Check sheet for the modelled part. Datum: model origin and axes. Units: mm. Give positions to 0.01 mm unless a question says otherwise; leave off trailing zeros. Loops run counter-clockwise (first coordinate to the right, second up) from the corner with the lowest first, then second, coordinate; pieces in that order, holes last. Notation, with made-up numbers: (-3, 83) -> (20, 83) arc R21 cw to (20, 121) -> close; hole circle Ø7 at (-35.5, -7). An arc over 180 degrees is marked (long way). Write each question's results on one line, items separated by ' | '. Start each with the question number.
1. Gauge pin test, flat ends, axial feed: pin 1 Ø1.4 at (y, z) = (37.5, 3) entering from -X; pin 2 Ø1.4 at (y, z) = (36, 2) entering from +X; pin 3 Ø1.4 at (x, z) = (157.5, 1.5) entering from -Y (3 decimals). Record the tip position at first contact, or that the pin passes through.
2. Cross-section at B-B on y = 34.5. Record the boundary of the cut face in (x, z).
3. Material ranges on L1, parallel to X at y = 16, z = 3.85; L2, parallel to Y at x = 154.5, z = 0.3; L3, parallel to X at y = 5, z = 2.5, recorded low to high. Write a range as from..to.
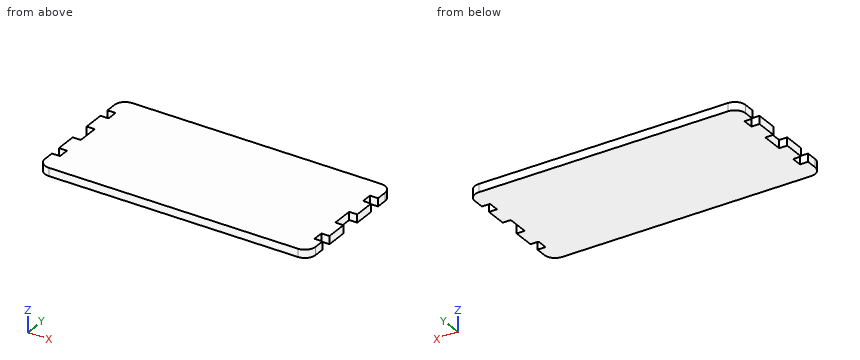
from build123d import *

# Parameters (mm, degrees)
F1_DEPTH = 4.7625


# Not quite as in the source:
# - a length typed as a fraction of an inch, garbled in the dataset ("3 / 203.2 mm" for 3/8 in), is restored
# - a feature names something its author has since deleted; it is built from what else it names


with BuildPart() as f1:
    # F0 (on Top) → F1 (new body)
    with BuildSketch(Plane.XY):
        with BuildLine():
            ThreePointArc((0, 6.35), (1.8598719395, 1.8598719395), (6.35, 0))
            Line((6.35, 0), (80.01, 0))
            Line((80.01, 0), (153.67, 0))
            ThreePointArc((153.67, 0), (158.1601280605, 1.8598719395), (160.02, 6.35))
            Line((160.02, 6.35), (160.02, 12.7))
            Line((160.02, 12.7), (155.2575, 12.7))
            Line((155.2575, 12.7), (155.2575, 19.05))
            Line((155.2575, 19.05), (160.02, 19.05))
            Line((160.02, 19.05), (160.02, 31.75))
            Line((160.02, 31.75), (155.2575, 31.75))
            Line((155.2575, 31.75), (155.2575, 44.45))
            Line((155.2575, 44.45), (160.02, 44.45))
            Line((160.02, 44.45), (160.02, 57.15))
            Line((160.02, 57.15), (155.2575, 57.15))
            Line((155.2575, 57.15), (155.2575, 63.5))
            Line((155.2575, 63.5), (160.02, 63.5))
            Line((160.02, 63.5), (160.02, 69.85))
            ThreePointArc((160.02, 69.85), (158.1601280605, 74.3401280605), (153.67, 76.2))
            Line((153.67, 76.2), (80.01, 76.2))
            Line((80.01, 76.2), (6.35, 76.2))
            ThreePointArc((6.35, 76.2), (1.8598719395, 74.3401280605), (0, 69.85))
            Line((0, 69.85), (0, 63.5))
            Line((0, 63.5), (4.7625, 63.5))
            Line((4.7625, 63.5), (4.7625, 57.15))
            Line((4.7625, 57.15), (0, 57.15))
            Line((0, 57.15), (0, 44.45))
            Line((0, 44.45), (4.7625, 44.45))
            Line((4.7625, 44.45), (4.7625, 31.75))
            Line((4.7625, 31.75), (0, 31.75))
            Line((0, 31.75), (0, 19.05))
            Line((0, 19.05), (4.7625, 19.05))
            Line((4.7625, 19.05), (4.7625, 12.7))
            Line((4.7625, 12.7), (0, 12.7))
            Line((0, 12.7), (0, 6.35))
        make_face()
    extrude(amount=F1_DEPTH)


solid = f1.part
Geometry says:
1) pin 1: x = 4.76 | pin 2: x = 155.26 | pin 3: y = 0.825
2) outline: (4.76, 0) -> (155.26, 0) -> (155.26, 4.76) -> (4.76, 4.76) -> close
3) L1: 4.76..155.26 | L2: 0.05..76.15 | L3: 0.15..159.87
